```python
from build123d import *

# Parameters (mm, degrees)
SKETCH_1_W      = 45
SKETCH_1_H      = 20
EXTRUDE_1_DEPTH = 1.6
SKETCH_2_R      = 8
EXTRUDE_2_DEPTH = 11.9
EXTRUDE_3_DEPTH = 3.4
SKETCH_4_W      = 10
SKETCH_4_H      = 2.5
EXTRUDE_4_DEPTH = 10


with BuildPart() as part:
    # 草图1 → 凸台-拉伸1 (new body)
    with BuildSketch(Plane(origin=(0, 0, 0), x_dir=(1, 0, 0), z_dir=(0, 1, 0))):
        Rectangle(SKETCH_1_W, SKETCH_1_H)
    extrude(amount=EXTRUDE_1_DEPTH)

    # 草图2 → 凸台-拉伸2 (add)
    with BuildSketch(Plane(origin=(0, 1.6, 0), x_dir=(1, 0, 0), z_dir=(0, 1, 0))):
        with Locations(Location((12.8, 0, 0), (0, 0, 90))):
            Circle(SKETCH_2_R)
        with Locations(Location((-12.8, 0, 0), (0, 0, 90))):
            Circle(SKETCH_2_R)
    extrude(amount=EXTRUDE_2_DEPTH)

    # 草图3 → 凸台-拉伸3 (add)
    with BuildSketch(Plane(origin=(0, 1.6, 0), x_dir=(1, 0, 0), z_dir=(0, 1, 0))):
        with BuildLine():
            Line((-3.25, -5.048754616), (3.25, -5.048754616))
            ThreePointArc((3.25, -5.048754616), (5, -6.798754616), (3.25, -8.548754616))
            Line((3.25, -8.548754616), (-3.25, -8.548754616))
            ThreePointArc((-3.25, -8.548754616), (-5, -6.798754616), (-3.25, -5.048754616))
        make_face()
    extrude(amount=EXTRUDE_3_DEPTH)

    # 草图4 → 凸台-拉伸4 (add)
    with BuildSketch(Plane.XZ):
        with Locations((0, -8.75)):
            Rectangle(SKETCH_4_W, SKETCH_4_H)
    extrude(amount=EXTRUDE_4_DEPTH)


solid = part.part
```
The model under review builds one solid part; all positions refer to its coordinate system, in mm. A direction names the side the tool comes from. Give positions to 0.01 mm unless a question says otherwise; leave off trailing zeros. Loops run counter-clockwise (first coordinate to the right, second up) from the corner with the lowest first, then second, coordinate; pieces in that order, holes last. Notation, with made-up numbers: (72, 60.5) - (131, 60.5) arc R34 cw to (131, 95.5) - close; hole circle Ø1 at (27, 45). An arc over 180 degrees is marked (long way). Answer as a JSON object with one key per item and string values.
Q1. To check wall thickness, follow line 1 along Y through (x, z) = (-20, 3.75); line 2 along X through (y, z) = (2.5, -0.25); line 3 along Z through (x, y) = (4.5, -3.5). State the ranges of each line that lie inside material, in increasing order.
Worked out:
{"line 1": "y = 0 to 1.6", "line 2": "x = -20.8 to -4.8, 4.8 to 20.8", "line 3": "z = -10 to -7.5"}
Q2. Add section A-A on x = 8. State the section outline as (y, z) points, plus the area to 3 significant figures.
Worked out:
{"outline": "(0, -10) - (1.6, -10) - (1.6, -6.4) - (13.5, -6.4) - (13.5, 6.4) - (1.6, 6.4) - (1.6, 10) - (0, 10) - close", "area": "184 mm^2"}
Q3. Add section B-B on z = 0. State the section outline as (x, y) points.
Worked out:
{"outline": "(-22.5, 0) - (22.5, 0) - (22.5, 1.6) - (20.8, 1.6) - (20.8, 13.5) - (4.8, 13.5) - (4.8, 1.6) - (-4.8, 1.6) - (-4.8, 13.5) - (-20.8, 13.5) - (-20.8, 1.6) - (-22.5, 1.6) - close"}
Q4. Insertion check: pin 1 (1.7 mm diameter, centred on x = 0, y = 4, fed in from +Z); pin 2 (5 mm diameter, centred on x = -3.5, z = -1.5, fed in from -Y); pin 3 (3 mm diameter, centred on x = -2.5, z = 6, fed in from +Y). Each pin has a flat end and moves straight along its axis. Give the tip position at first contact, or say it passes through.
Worked out:
{"pin 1": "stops at z = 8.55", "pin 2": "stops at y = 0", "pin 3": "stops at y = 5"}
Q5. Add section D-D on x = 12.8. State the section outline as (y, z) points.
Worked out:
{"outline": "(0, -10) - (1.6, -10) - (1.6, -8) - (13.5, -8) - (13.5, 8) - (1.6, 8) - (1.6, 10) - (0, 10) - close"}
Q6. Add section C-C on y = -6.75. State the section outline as (x, z) points, plus the area to 3 significant figures.
Worked out:
{"outline": "(-5, -10) - (5, -10) - (5, -7.5) - (-5, -7.5) - close", "area": "25.0 mm^2"}
Q7. For faces 1 (the flat face through (0, -5, -7.5)), 2 (the flat face through (5, -5, -9)), 3 (the flat face through (0, 3, 8.549)), 4 (the cylindrical face through (5, 3.3, 6.8)), list the 3-axis set-ups (+Z, -Z, +X, -X, +Y, -Y) from which the entire face can be reached by the end or side of a thin tool; tool diameter is ignored.
Worked out:
{"face 1": "+Z, +X, -X, -Y", "face 2": "+Z, -Z, +X, -Y", "face 3": "+Z, +X, -X, +Y", "face 4": "+Y"}
